Part model, mm, in its own coordinate system. A direction names the side the tool comes from. Coordinates: 2 decimals unless noted, no trailing zeros. Order: outer loops, then holes, each group sorted by start corner. A loop starts at its lowest first (then second) coordinate and runs counter-clockwise, first axis right, second up. Notation, with made-up numbers: (12, 10.25) - (68, 10.25) arc R21 cw to (68, 46.25) - close; hole circle Ø11 at (-18, 11.5). An arc over 180 degrees is marked (long way). Use a Markdown table: item, result. Add a question column.
1) Tool access for faces 5 (the face through (11.5, 0.2, 0.7)), 6 (the face through (-17.9, -5, 0.7)): list every direction of +Z, -Z, +X, -X, +Y, -Y with a clear straight run to the whole face (end or side of a thin tool).
2) Saw through at A-A on z = 0.6. List the corners of the cut face in (x, y), then the cut area to 3 significant figures.
3) Saw through at B-B on y = 0. List the corners of the cut face in (x, z).
4) Saw through at D-D on x = -12.5. List the corners of the cut face in (y, z).
5) Wall check: L1, parallel to Y at x = -21.5, z = 0.45; L2, parallel to X at y = -2, z = 0.85; L3, parallel to X at y = -3, z = 0.55. Give the ranges that are in metal, low to high. Write a range as [from, to].
6) Two-plate mould, pull along Y, no slides. Class faces 1 (the face through (-20, -6.05, 1)), 2 (the face through (-23, 16, 1)), 3 (the face through (-24, 0, 1)), 4 (the face through (-9.301, -13.604, 0.74)): +Y half, -Y half, draft (parallel to the pull), parting line (faces both ways), or undercut.
7) Saw through at C-C on x = 0. List the corners of the cut face in (y, z), then the cut area to 3 significant figures.
8) Drop flat-ended pins along their axis: P1, Ø0.8, axis at x = -20, z = 1, coming from the +Y side; P2, Ø9, axis at x = 0, y = 0, coming from the +Z side. Give the stop position or say it passes through.
Autodesk Inventor part; units mm, degrees
ref_plane "YZ Plane" through (0, 0, 0) normal (1, 0, 0) x (0, 1, 0)
ref_plane "XZ Plane" through (0, 0, 0) normal (0, 1, 0) x (-1, 0, 0)
ref_plane "XY Plane" through (0, 0, 0) normal (0, 0, 1) x (1, 0, 0)
sketch "スケッチ1" plane through (0, 0, 0) normal (0, 0, 1) x (1, 0, 0)
  circle A0 centre (0, 0) radius 10.5 construction
  line L0 (-12, 10.583) -> (-12, -10.583) construction
  arc A1 (0, 16) -> (-12, 10.583) centre (0, 0) ccw construction
  line L1 (0, 16) -> (33.5167, 16) construction
  line L2 (33.5167, 16) -> (33.5167, -16) construction
  line L3 (33.5167, -16) -> (0, -16) construction
  arc A2 (-12, -10.583) -> (0, -16) centre (0, 0) ccw construction
  circle A3 centre (0, 8.5) radius 1.35
  circle A4 centre (-8.5, 0) radius 1.35
  circle A5 centre (0, -8.5) radius 1.35
  circle A6 centre (8.5, 0) radius 1.35
  circle A7 centre (0, 0) radius 5.05
  circle A8 centre (0, 0) radius 16 construction
  line L4 (-21.5, 6) -> (-19, 6) construction
  line L5 (-19, 6) -> (-19, -6) construction
  line L6 (-19, -6) -> (-21.5, -6) construction
  line L7 (-21.5, -6) -> (-21.5, 6) construction
  circle A9 centre (0, 0) radius 19 construction
  line L8 (-18.95, 6.05) -> (-21.55, 6.05) construction
  line L9 (-21.55, 6.05) -> (-21.55, -6.05) construction
  line L10 (-21.55, -6.05) -> (-18.95, -6.05) construction
  line L11 (-18.95, -6.05) -> (-18.95, 6.05) construction
  circle A10 centre (-21.55, 5) radius 1.05 construction
  line L12 (-18.95, 6.05) -> (-21.55, 6.05)
  arc A11 (-21.55, 6.05) -> (-21.55, 3.95) centre (-21.55, 5) ccw
  line L13 (-21.55, 3.95) -> (-21.55, -3.95)
  line L14 (-20.25, 6.05) -> (-20.25, -6.05) construction
  line L15 (-21.55, 0) -> (-19, 0) construction
  arc A12 (-21.55, -3.95) -> (-21.55, -6.05) centre (-21.55, -5) ccw
  line L16 (-21.55, -6.05) -> (-18.95, -6.05)
  line L17 (-18.95, 3.95) -> (-18.95, -3.95)
  arc A13 (-18.95, 3.95) -> (-18.95, 6.05) centre (-18.95, 5) ccw
  arc A14 (-18.95, -6.05) -> (-18.95, -3.95) centre (-18.95, -5) ccw
  line L18 (-24, 6) -> (-24, -6)
  circle A15 centre (-21.5, 13) radius 1.55
  circle A16 centre (-21.5, -13) radius 1.55
  line L19 (-24, 16) -> (-21.201, 16)
  line L20 (-24, -16) -> (-21.201, -16)
  arc A17 (2.2701, -11.2737) -> (2.2701, 11.2737) centre (0, 0) ccw
  line L21 (-24, 16) -> (-24, 6)
  circle A18 centre (-21.5, 13) radius 3 construction
  line L22 (-24, -16) -> (-24, -6)
  line L23 (-21.201, 16) -> (2.2701, 11.2737)
  line L24 (2.2701, -11.2737) -> (-21.201, -16)
  point P0 (-12, 0)
  point P1 (-20.275, 0)
  dimension "d29" = 2.1
  dimension "d0" = 21
  dimension "d1" = 16
  dimension "d2" = 12
  dimension "d3" = 8.5
  dimension "d4" = 2.7
  dimension "d7" = 360
  dimension "d9" = 10.1
  dimension "d10" = 2.5
  dimension "d11" = 3
  dimension "d27" = 10
  dimension "d30" = 0.05
  dimension "d31" = 7
  dimension "d33" = 3.1
  dimension "d41" = 2.5
  dimension "d43" = 1
extrude "押し出し1" add sketch "スケッチ1" along normal blind 1.5
sketch "スケッチ2" plane through (0, 0, 0) normal (0, 0, -1) x (-1, 0, 0)
  circle A0 centre (0, -8.5) radius 1.35
  circle A1 centre (0, -8.5) radius 1.35
  circle A2 centre (-8.5, 0) radius 1.35
  circle A3 centre (-8.5, 0) radius 1.35
  circle A4 centre (8.5, 0) radius 1.35
  circle A5 centre (8.5, 0) radius 1.35
  circle A6 centre (21.5, -13) radius 1.55
  circle A7 centre (21.5, -13) radius 1.55
  circle A8 centre (0, 8.5) radius 1.35
  circle A9 centre (0, 8.5) radius 1.35
  circle A10 centre (21.5, 13) radius 1.55
  circle A11 centre (21.5, 13) radius 1.55
  point P0 (0, 0)
extrude "押し出し2" add sketch "スケッチ2" against normal up to surface (1.5 mm away)
equation "\"d27\" = d21"
equation "\"d31\" = d23"
properties part number "肩_サブフレーム_1_1" material "GFRP"
Results are:
| question | item | result |
|---|---|---|
| 1 | face 5 | +Z, -Z, +X |
| 1 | face 6 | +Z, -Z |
| 2 | outline | (-24, -16) - (-21.2, -16) - (2.27, -11.27) arc R11.5 ccw to (2.27, 11.27) - (-21.2, 16) - (-24, 16) - close; hole (-21.55, -6.05) - (-18.95, -6.05) arc R1.05 ccw to (-18.95, -3.95) - (-18.95, 3.95) arc R1.05 ccw to (-18.95, 6.05) - (-21.55, 6.05) arc R1.05 ccw to (-21.55, 3.95) - (-21.55, -3.95) arc R1.05 ccw to start; hole circle Ø10.1 at (0, 0) |
| 2 | area | 767 mm2 |
| 3 | outline | (-24, 0) - (-21.55, 0) - (-21.55, 1.5) - (-24, 1.5) - close; (-18.95, 0) - (-5.05, 0) - (-5.05, 1.5) - (-18.95, 1.5) - close; (5.05, 0) - (11.5, 0) - (11.5, 1.5) - (5.05, 1.5) - close |
| 4 | outline | (-14.25, 0) - (14.25, 0) - (14.25, 1.5) - (-14.25, 1.5) - close |
| 5 | L1 | [-16, -6.05], [6.05, 16] |
| 5 | L2 | [-24, -21.55], [-18.95, -4.64], [4.64, 11.32] |
| 5 | L3 | [-24, -21.55], [-18.95, -4.06], [4.06, 11.1] |
| 6 | face 1 | undercut |
| 6 | face 2 | +Y half |
| 6 | face 3 | draft |
| 6 | face 4 | -Y half |
| 7 | outline | (-11.73, 0) - (-5.05, 0) - (-5.05, 1.5) - (-11.73, 1.5) - close; (5.05, 0) - (11.73, 0) - (11.73, 1.5) - (5.05, 1.5) - close |
| 7 | area | 20.0 mm2 |
| 8 | P1 | y = 15.84 |
| 8 | P2 | through |
